Read the model definition and answer for the solid it produces. Units are mm, in the model's axes. Face numbers are marked on the shaded views. A direction names the side the tool comes from. Coordinates: 2 decimals unless noted, no trailing zeros. Write each loop counter-clockwise with the first axis right and the second up, starting at its lowest first coordinate (ties: lowest second). Pieces come first, ordered by that corner, then holes.
(1) The part is cut by section D-D, the plane x = 4.25. Determine the outline of the cut face in (y, z), and give its area (3 significant figures).
(2) The part is cut by section C-C, the plane z = 7.5. Determine the outline of the cut face in (x, y).
(3) Straight lines are drawn through the part: line 1 along Z through (x, y) = (5.25, 12.7); line 2 along Y through (x, z) = (4.75, 6.35); line 3 along Y through (x, z) = (14.5, 10). For each, find the intervals that lie inside material, in ascending order.
(4) Determine the mould class of the marked faces 1, 2, 3 and 4 for opening direction Z: pulls with the +Z half, pulls with the -Z half, needs draft (parallel to the pull), parting line crosses it, or undercut.
(5) Given pin 1 (5 mm diameter, centred on x = 11.5, z = 7, fed in from +Y); pin 2 (1 mm diameter, centred on y = 15, z = 5.5, fed in from +X); pin 3 (3 mm diameter, centred on y = 12.7, z = 6.35, fed in from -X), each flat-ended and moving along its own axis, determine where each tip first touches the part or whether it passes through.
(6) Which of the six approach directions +Z, -Z, +X, -X, +Y, -Y give full straight-line access (tool end or side, diameter ignored) to the marked faces 5 and 6?
(7) The part is cut by section A-A, the plane x = 12.7. Determine the outline of the cut face in (y, z).
```python
from build123d import *

# Parameters (mm, degrees)
BOSS_EXTRUDE1_DEPTH                        = 12.7
F_13_64_0_20313_DIAMETER_HOLE1_D           = 5.159502
F_13_64_0_20313_DIAMETER_HOLE1_ON_FACE_2_D = 5.159502


with BuildPart() as part:
    # Sketch1 → Boss-Extrude1 (new body)
    with BuildSketch(Plane.XY):
        Polygon((0, 0), (11.162631579, 0), (19.05, 0), (19.05, 6.35), (6.35, 6.35), (6.35, 19.05), (0, 19.05), align=None)
    extrude(amount=BOSS_EXTRUDE1_DEPTH)

    # 13/64 (0.20313) Diameter Hole1 (through all)
    with Locations(Plane(origin=(6.35, 12.7, 6.35), x_dir=(0, 0, 1), z_dir=(1, 0, 0))):
        with Locations((0, 0)):
            Hole(F_13_64_0_20313_DIAMETER_HOLE1_D / 2)

    # 13/64 (0.20313) Diameter Hole1 on face 2 (through all)
    with Locations(Plane(origin=(12.7, 6.35, 6.35), x_dir=(0, 0, 1), z_dir=(0, 1, 0))):
        with Locations((0, 0)):
            Hole(F_13_64_0_20313_DIAMETER_HOLE1_ON_FACE_2_D / 2)


solid = part.part
```
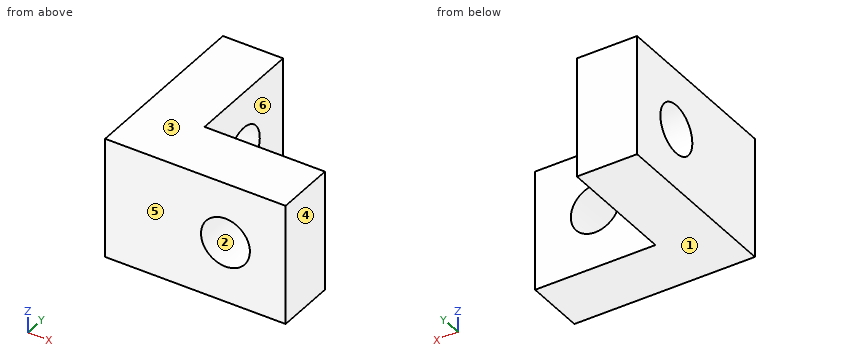
Computed:
1. outline: (0, 0) - (19.05, 0) - (19.05, 12.7) - (0, 12.7) - close; hole circle Ø5.16 at (12.7, 6.35)
1. area: 221 mm2
2. outline: (0, 0) - (10.39, 0) - (10.39, 6.35) - (6.35, 6.35) - (6.35, 10.39) - (0, 10.39) - close; (0, 15.01) - (6.35, 15.01) - (6.35, 19.05) - (0, 19.05) - close; (15.01, 0) - (19.05, 0) - (19.05, 6.35) - (15.01, 6.35) - close
3. line 1: z = 0 to 3.77, 8.93 to 12.7
3. line 2: y = 0 to 10.12, 15.28 to 19.05
3. line 3: y = 0 to 6.35
4. face 1: pulls with the -Z half
4. face 2: undercut
4. face 3: pulls with the +Z half
4. face 4: needs draft
5. pin 1: stops at y = 6.35
5. pin 2: stops at x = 6.35
5. pin 3: passes through
6. face 5: +Z, -Z, +X, -X, -Y
6. face 6: +Z, -Z, +X, +Y
7. outline: (0, 0) - (6.35, 0) - (6.35, 3.77) - (0, 3.77) - close; (0, 8.93) - (6.35, 8.93) - (6.35, 12.7) - (0, 12.7) - close
